Verification items for the finished model (mm, model axes). Coordinates: 2 decimals unless noted, no trailing zeros. Order: outer loops, then holes, each group sorted by start corner. A loop starts at its lowest first (then second) coordinate and runs counter-clockwise, first axis right, second up. Notation, with made-up numbers: M 78,-24.75 L 118,-24.75 A19 cw 118,-10.75 Z; hole C -2,83 d4. An arc over 180 degrees is marked long. Answer as a JSON object with one key per item and string values. Group by question number.
(1) Material ranges on line 1 (Y direction, x = -4.09, z = 3.35); line 2 (X direction, y = -60, z = 1.3); line 3 (X direction, y = 75, z = 1.85), recorded low to high.
(2) Cross-section at D-D (z = 1.5). Count the separate pieces of the cut face and the enclosed holes in it, plus the area to 3 significant figures.
(3) Gauge pin test, flat ends, axial feed: pin 1 Ø1.1 at (y, z) = (52.5, 3.5) entering from -X; pin 2 Ø2.5 at (x, z) = (-62.5, 4.5) entering from +Y; pin 3 Ø1 at (y, z) = (-10.5, 1) entering from +X. Record the tip position at first contact, or that the pin passes through.
(4) Cross-section at B-B (y = -0.5). Enter the section's corners in (x, z).
(5) Cross-section at A-A (x = 69). Enter the section's corners in (y, z), plus the area to 3 significant figures.
(6) Cross-section at C-C (x = -45). Enter the section's corners in (y, z).
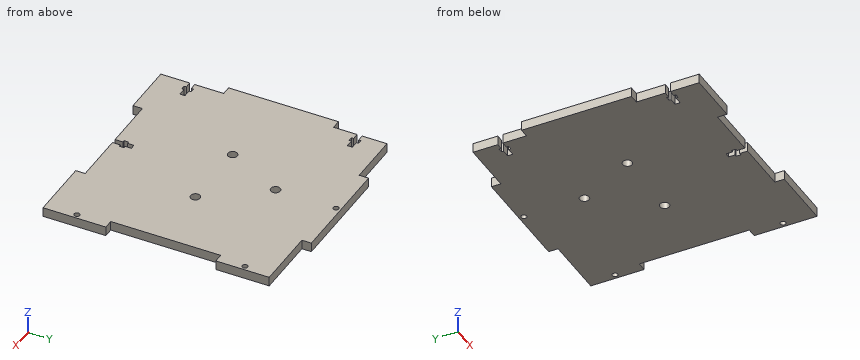
from build123d import *

# Parameters (mm, degrees)
SKETCH1_R           = 1.75
BOSS_EXTRUDE2_DEPTH = 6
SKETCH3_R           = 3
CUT_EXTRUDE1_DEPTH  = 7
SKETCH4_R           = 3
CUT_EXTRUDE2_DEPTH  = 7


with BuildPart() as part:
    # Sketch1 → Boss-Extrude2 (new body)
    with BuildSketch(Plane.XY):
        Polygon((72, 72), (32, 72), (32, 78), (-38, 78), (-38, 72), (-72, 72), (-72, 56.2), (-67.772810154, 56.2), (-67.772810154, 57.6), (-64.957983727, 57.6), (-64.957983727, 56.2), (-60, 56.2), (-60, 53), (-64.957983727, 53), (-64.957983727, 51.568504207), (-67.772810154, 51.568504207), (-67.772810154, 53), (-72, 53), (-72, 38), (-78, 38), (-78, -32), (-72, -32), (-72, -50.4), (-67.78187279, -50.4), (-67.78187279, -49), (-64.967046362, -49), (-64.967046362, -50.4), (-60, -50.4), (-60, -53.6), (-64.967046362, -53.6), (-64.967046362, -55), (-67.78187279, -55), (-67.78187279, -53.6), (-72, -53.6), (-72, -72), (-38, -72), (-38, -66), (-4.6, -66), (-4.6, -61), (-6, -61), (-6, -58), (-4.6, -58), (-4.6, -54), (-1.4, -54), (-1.4, -58), (0, -58), (0, -61), (-1.4, -61), (-1.4, -66), (32, -66), (32, -72), (72, -72), (72, -32), (66, -32), (66, 38), (72, 38), align=None)
        with Locations((69, -52)):
            Circle(SKETCH1_R, mode=Mode.SUBTRACT)
        with Locations((69, 55)):
            Circle(SKETCH1_R, mode=Mode.SUBTRACT)
        with Locations((-4.09, 75)):
            Circle(SKETCH1_R, mode=Mode.SUBTRACT)
    extrude(amount=BOSS_EXTRUDE2_DEPTH)

    # Sketch3 → Cut-Extrude1 (cut, through all)
    with BuildSketch(Plane(origin=(0, 0, 0), x_dir=(-1, 0, 0), z_dir=(0, 0, -1))):
        with Locations((3.924742841, 36.491728523)):
            Circle(SKETCH3_R)
    extrude(amount=-CUT_EXTRUDE1_DEPTH, mode=Mode.SUBTRACT)

    # Sketch4 → Cut-Extrude2 (cut, through all)
    with BuildSketch(Plane(origin=(0, 0, 0), x_dir=(-1, 0, 0), z_dir=(0, 0, -1))):
        with Locations((-23, -0.5)):
            Circle(SKETCH4_R)
        with Locations((22.5, -0.5)):
            Circle(SKETCH4_R)
    extrude(amount=-CUT_EXTRUDE2_DEPTH, mode=Mode.SUBTRACT)


solid = part.part
Taken from the geometry:
{
 "1": {"line 1": "y = -54 to 33.5, 39.49 to 73.25, 76.75 to 78", "line 2": "x = -72 to -6, 0 to 72", "line 3": "x = -38 to -5.84, -2.34 to 32"},
 "2": {"separate pieces": "1", "enclosed holes": "6", "area": "20,500 mm²"},
 "3": {"pin 1": "stops at x = -72", "pin 2": "stops at y = 72", "pin 3": "stops at x = 66"},
 "4": {"outline": "M -78,0 L -25.5,0 L -25.5,6 L -78,6 Z; M -19.5,0 L 20,0 L 20,6 L -19.5,6 Z; M 26,0 L 66,0 L 66,6 L 26,6 Z"},
 "5": {"outline": "M -72,0 L -53.75,0 L -53.75,6 L -72,6 Z; M -50.25,0 L -32,0 L -32,6 L -50.25,6 Z; M 38,0 L 53.25,0 L 53.25,6 L 38,6 Z; M 56.75,0 L 72,0 L 72,6 L 56.75,6 Z", "area": "402 mm²"},
 "6": {"outline": "M -72,0 L 72,0 L 72,6 L -72,6 Z"}
}
